Design review of the part shown in the three views and the two pictorial views. Dimensions are in mm from the part's minimum x, y and z. Coordinates: 2 decimals unless noted, no trailing zeros. Order: outer loops, then holes, each group sorted by start corner. A loop starts at its lowest first (then second) coordinate and runs counter-clockwise, first axis right, second up. Notation, with made-up numbers: (-23.5, -36.5) -> (-8.5, -36.5) arc R18 cw to (-8.5, -24.5) -> close; hole circle Ø10 at (53, 57). An arc over 180 degrees is marked (long way). Write item = value, one per line. Start each with the question number.
1) Consider section B-B on z = 144.5. Give the boundary of the cut face in (x, y).
2) Wall thickness on probe 1 along Y at (x, z) = (127, 191); probe 2 along Z at (x, y) = (87, 130); probe 3 along X at (y, z) = (38, 77): over which ranges is each line inside the solid? List them lowest first. Write a range as [from, to].
3) Consider section A-A on x = 127. Give the boundary of the cut face in (y, z), and give its area (3 significant figures).
4) Insertion check: pin 1 Ø6 at (x, z) = (191, 205.5) entering from -Y; pin 2 Ø5 at (x, y) = (158.5, 183.5) entering from +Z; pin 3 Ø1.5 at (x, z) = (200, 175) entering from -Y. Each pin has a flat end and moves straight along its axis. Give the tip position at first contact, or say it passes through.
5) Draft analysis for pull direction X (two halves, no side actions). For the marked faces 1, 2 and 3, state which applies: +X half, -X half, draft (parallel to the pull), parting line (faces both ways), or undercut.
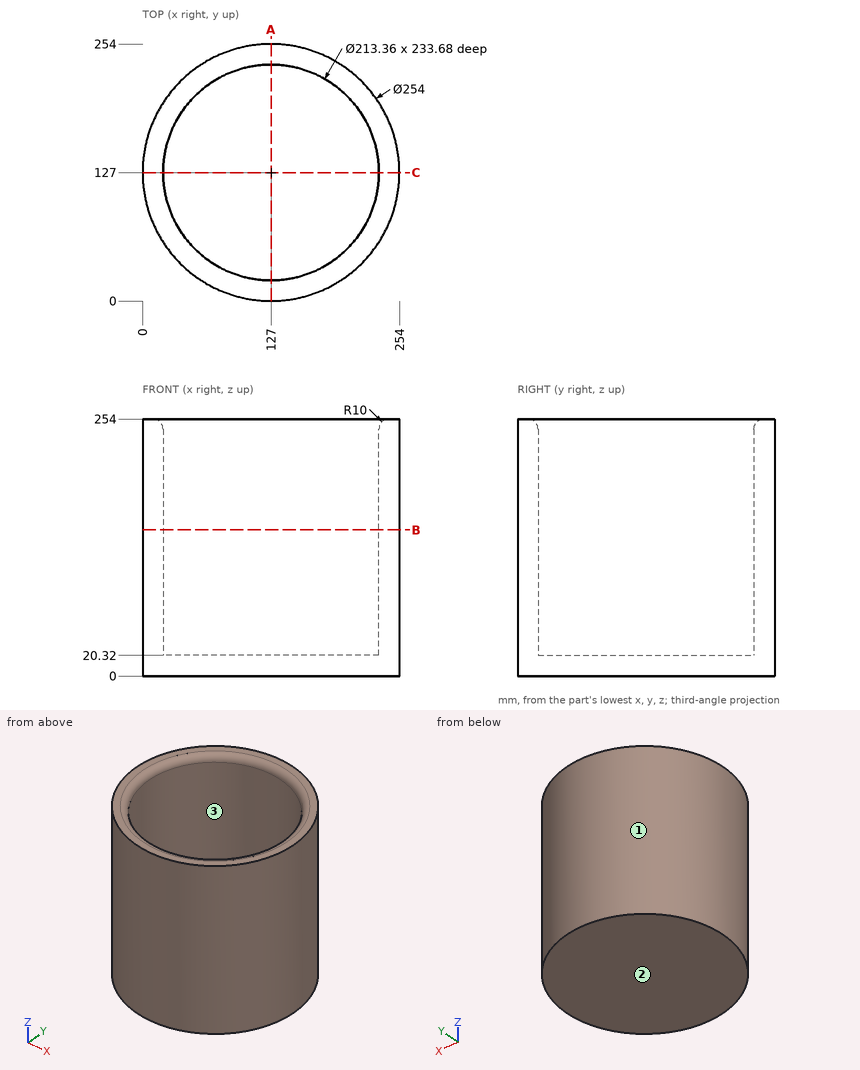
Answer sheet:
q1.outline = circle Ø254 at (127, 127); hole circle Ø213.36 at (127, 127)
q2.probe_1 = [0, 20.32], [233.68, 254]
q2.probe_2 = [0, 20.32]
q2.probe_3 = [36.4, 68.18], [185.82, 217.6]
q3.outline = (0, 0) -> (254, 0) -> (254, 254) -> (243.68, 254) arc R10 ccw to (233.68, 244) -> (233.68, 20.32) -> (20.32, 20.32) -> (20.32, 244) arc R10 ccw to (10.32, 254) -> (0, 254) -> close
q3.area = 14,600 mm2
q4.pin_1 = 15.61
q4.pin_2 = 20.32
q4.pin_3 = 22.55
q5.face_1 = parting line
q5.face_2 = draft
q5.face_3 = undercut
